Geometry: see drawing. Coordinates: mm, zero at the bounding-box minimum. A direction names the side the tool comes from. Round coordinates to 2 decimals unless told otherwise and drop trailing zeros. Loops run counter-clockwise (first coordinate to the right, second up) from the corner with the lowest first, then second, coordinate; pieces in that order, holes last.
(1) Access query for the marked faces 1, 2 and 3. Directions: +Z, -Z, +X, -X, +Y, -Y. A direction counts if a zero-diameter tool reaches every point of the face in a straight line with its end or side. Return the directions, or none.
(2) Cut plane C-C, the plane z = 3.3. Output: boundary loops of the cut face in (x, y), and give its area (3 significant figures).
(3) Line query: line 1 (Y direction, x = 41.5, z = 1.65); line 2 (Y direction, x = 26.85, z = 3.75); line 3 (Y direction, x = 16.5, z = 1.1). Output: solid intervals per line, ascending.
(4) Cut plane B-B, the plane y = 15.7. Output: boundary loops of the cut face in (x, z).
(5) Cut plane A-A, the plane x = 41.5. Output: boundary loops of the cut face in (y, z).
(6) First-contact query: pin 1 Ø0.5 at (x, y) = (27, 15.5) entering from +Z; pin 2 Ø1.5 at (x, z) = (14.5, 3) entering from -Y. Flat tips, straight axial feed; report the tip coordinate or a pass-through.
(7) Cut plane D-D, the plane z = 1. Output: boundary loops of the cut face in (x, y), and give its area (3 significant figures).
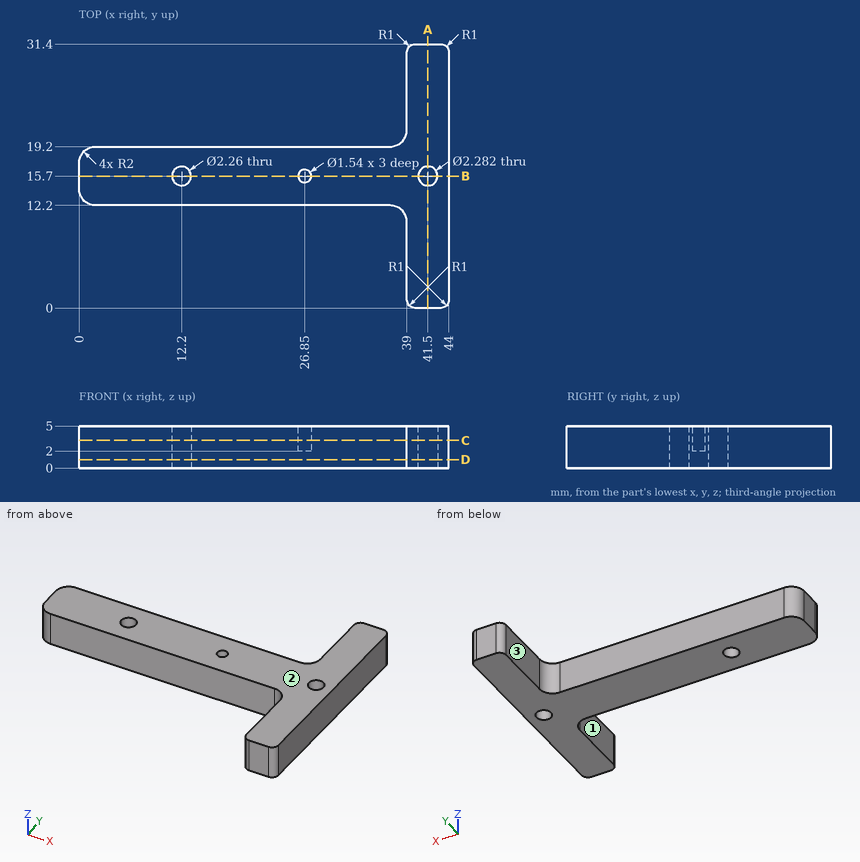
Reported:
1. face 1: +Z, -Z, -X, -Y
1. face 2: +Z, +X, -X, +Y, -Y
1. face 3: +Z, -Z, -X, +Y
2. outline: (0, 14.2) arc R2 ccw to (2, 12.2) - (37, 12.2) arc R2 cw to (39, 10.2) - (39, 1) arc R1 ccw to (40, 0) - (43, 0) arc R1 ccw to (44, 1) - (44, 30.4) arc R1 ccw to (43, 31.4) - (40, 31.4) arc R1 ccw to (39, 30.4) - (39, 21.2) arc R2 cw to (37, 19.2) - (2, 19.2) arc R2 ccw to (0, 17.2) - close; hole circle Ø2.26 at (12.2, 15.7); hole circle Ø1.54 at (26.85, 15.7); hole circle Ø2.28 at (41.5, 15.7)
2. area: 419 mm2
3. line 1: y = 0 to 14.56, 16.84 to 31.4
3. line 2: y = 12.2 to 14.93, 16.47 to 19.2
3. line 3: y = 12.2 to 19.2
4. outline: (0, 0) - (11.07, 0) - (11.07, 5) - (0, 5) - close; (13.33, 0) - (40.36, 0) - (40.36, 5) - (27.62, 5) - (27.62, 2) - (26.08, 2) - (26.08, 5) - (13.33, 5) - close; (42.64, 0) - (44, 0) - (44, 5) - (42.64, 5) - close
5. outline: (0, 0) - (14.56, 0) - (14.56, 5) - (0, 5) - close; (16.84, 0) - (31.4, 0) - (31.4, 5) - (16.84, 5) - close
6. pin 1: stops at z = 2
6. pin 2: stops at y = 12.2
7. outline: (0, 14.2) arc R2 ccw to (2, 12.2) - (37, 12.2) arc R2 cw to (39, 10.2) - (39, 1) arc R1 ccw to (40, 0) - (43, 0) arc R1 ccw to (44, 1) - (44, 30.4) arc R1 ccw to (43, 31.4) - (40, 31.4) arc R1 ccw to (39, 30.4) - (39, 21.2) arc R2 cw to (37, 19.2) - (2, 19.2) arc R2 ccw to (0, 17.2) - close; hole circle Ø2.26 at (12.2, 15.7); hole circle Ø2.28 at (41.5, 15.7)
7. area: 421 mm2
